Could you check a few things on this model? Use its own coordinates, in mm. Face numbers are marked on the shaded views. A direction names the side the tool comes from. Give positions to 0.01 mm unless a question says otherwise; leave off trailing zeros. Loops run counter-clockwise (first coordinate to the right, second up) from the corner with the lowest first, then second, coordinate; pieces in that order, holes last. Notation, with made-up numbers: M 23.25,48.25 L 69.25,48.25 A16 cw 69.25,53.25 Z; hole C 69,-27.5 d11. An arc over 180 degrees is marked long. Use a Markdown table: item, result. Add a question column.
1) Suppose I cut it at C-C on y = 9.5. List the corners of the cut face in (x, z) for me (3 decimals).
2) If I drill on line 1 along Y through (x, z) = (-15, 13.5) (3 decimals); line 2 along X through (y, z) = (25.55, 8.5) (3 decimals); line 3 along Y through (x, z) = (6, 6) (3 decimals), over which ranges is the centre line in solid material (lowest first)? Write a range as [from, to].
3) Suppose I cut it at B-B on x = -18.5. List the corners of the cut face in (y, z) for me (3 decimals).
4) Will this pin go through, and if not, where does the flat tip stop? pin 1 Ø4 at (x, y) = (-5.2, 25.55) entering from -Z.
5) Suppose I cut it at A-A on z = 2.25. Count the separate pieces of the cut face and the enclosed holes in it, and give its area (3 significant figures).
6) Which directions (+Z, -Z, +X, -X, +Y, -Y) give clear straight access to the entire face, cutting with the end or side of a thin tool? Please do the marked faces 1 and 2.
7) Suppose I cut it at D-D on x = -5.2. List the corners of the cut face in (y, z) for me (3 decimals).
8) We'd pull the mould along Y, two halves only. Please class the marked faces 3, 4, 5 and 6: +Y half, -Y half, draft (parallel to the pull), parting line (faces both ways), or undercut.
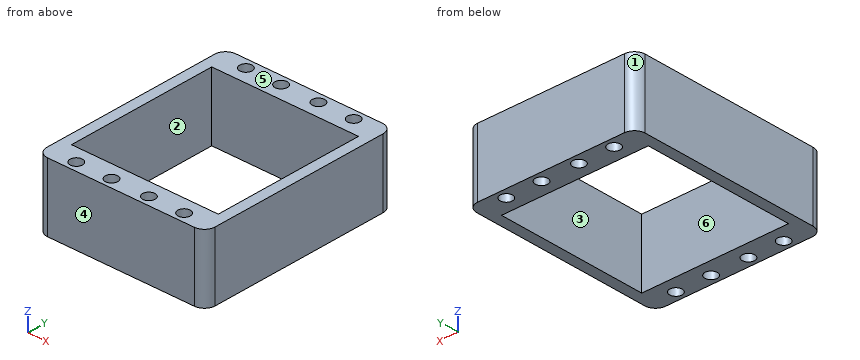
```python
from build123d import *

# Parameters (mm, degrees)
SKETCH1_W           = 46.85
SKETCH1_H           = 56.6
SKETCH1_R           = 1.725
SKETCH1_W_2         = 40.85
SKETCH1_H_2         = 42.25
BOSS_EXTRUDE1_DEPTH = 18.8
FILLET1_R           = 3


with BuildPart() as part:
    # Sketch1 → Boss-Extrude1 (new body)
    with BuildSketch(Plane.XY):
        Rectangle(SKETCH1_W, SKETCH1_H)
        with Locations((-15, -25.55)):
            Circle(SKETCH1_R, mode=Mode.SUBTRACT)
        with Locations((-5.2, -25.55)):
            Circle(SKETCH1_R, mode=Mode.SUBTRACT)
        with Locations((5.2, -25.55)):
            Circle(SKETCH1_R, mode=Mode.SUBTRACT)
        with Locations((15, -25.55)):
            Circle(SKETCH1_R, mode=Mode.SUBTRACT)
        with Locations(Location((15, 25.55, 0), (0, 0, 180))):
            Circle(SKETCH1_R, mode=Mode.SUBTRACT)
        with Locations(Location((5.2, 25.55, 0), (0, 0, 180))):
            Circle(SKETCH1_R, mode=Mode.SUBTRACT)
        with Locations(Location((-5.2, 25.55, 0), (0, 0, 180))):
            Circle(SKETCH1_R, mode=Mode.SUBTRACT)
        with Locations(Location((-15, 25.55, 0), (0, 0, 180))):
            Circle(SKETCH1_R, mode=Mode.SUBTRACT)
        Rectangle(SKETCH1_W_2, SKETCH1_H_2, mode=Mode.SUBTRACT)
    extrude(amount=BOSS_EXTRUDE1_DEPTH)

    # Fillet1
    fillet1_edges = [part.edges().sort_by_distance(p)[0] for p in [
        (-23.425, 28.3, 9.4),
        (23.425, 28.3, 9.4),
        (23.425, -28.3, 9.4),
        (-23.425, -28.3, 9.4),
    ]]
    fillet(fillet1_edges, radius=FILLET1_R)


solid = part.part
```
Answer block:
| question | item | result |
|---|---|---|
| 1 | outline | M -23.425,0 L -20.425,0 L -20.425,18.8 L -23.425,18.8 Z; M 20.425,0 L 23.425,0 L 23.425,18.8 L 20.425,18.8 Z |
| 2 | line 1 | y = [-28.3, -27.275], [-23.825, -21.125], [21.125, 23.825], [27.275, 28.3] |
| 2 | line 2 | x = [-23.415, -16.725], [-13.275, -6.925], [-3.475, 3.475], [6.925, 13.275], [16.725, 23.415] |
| 2 | line 3 | y = [-28.3, -27.078], [-24.022, -21.125], [21.125, 24.022], [27.078, 28.3] |
| 3 | outline | M -28.3,0 L -21.125,0 L -21.125,18.8 L -28.3,18.8 Z; M 21.125,0 L 28.3,0 L 28.3,18.8 L 21.125,18.8 Z |
| 4 | pin 1 | stops at z = 0 |
| 5 | separate pieces | 1 |
| 5 | enclosed holes | 9 |
| 5 | area | 843 mm^2 |
| 6 | face 1 | +Z, -Z, -X, +Y |
| 6 | face 2 | +Z, -Z |
| 7 | outline | M -28.3,0 L -27.275,0 L -27.275,18.8 L -28.3,18.8 Z; M -23.825,0 L -21.125,0 L -21.125,18.8 L -23.825,18.8 Z; M 21.125,0 L 23.825,0 L 23.825,18.8 L 21.125,18.8 Z; M 27.275,0 L 28.3,0 L 28.3,18.8 L 27.275,18.8 Z |
| 8 | face 3 | undercut |
| 8 | face 4 | -Y half |
| 8 | face 5 | draft |
| 8 | face 6 | undercut |
